Geometry check sheet. Reference: drawing and pictorial views, mm from the part's lowest x, y, z. A direction names the side the tool comes from. Round coordinates to 2 decimals unless told otherwise and drop trailing zeros. Write each loop counter-clockwise with the first axis right and the second up, starting at its lowest first coordinate (ties: lowest second). Pieces come first, ordered by that corner, then holes. Notation, with made-up numbers: M 32.25,-22.5 L 48.25,-22.5 A19 cw 48.25,3.5 Z; hole C -38.75,-30.75 d4. An arc over 180 degrees is marked long. Answer in a Markdown table with one row per item. Add a question column.
1. Sectioned sample at A-A on z = 18. Record the cut outline in (x, y).
2. Sectioned sample at B-B on y = 7.5. Record the cut outline in (x, z).
3. Sectioned sample at D-D on x = 38.5. Record the cut outline in (y, z).
4. Material ranges on probe 1 along Y at (x, z) = (37.5, 42.1); probe 2 along X at (y, z) = (7, 43.5) (1 decimal); probe 3 along Z at (x, y) = (29.5, 3.5), recorded low to high.
5. Go/stop test with flat-tipped pins: pin 1 Ø5.5 at (x, y) = (37.5, 7.5) entering from +Z; pin 2 Ø12 at (x, y) = (31.5, 21.5) entering from -Z; pin 3 Ø3 at (x, z) = (15, 31.5) entering from -Y; pin 4 Ø3 at (y, z) = (37.5, 14) entering from -X (1 decimal). Record where each tip stops, or that it passes through.
6. Draft check along X on the marked faces 1, 2 and 3. Enter one of: pulls with the +X half, pulls with the -X half, needs draft (parallel to the pull), parting line crosses it, or undercut.
7. Sectioned sample at C-C on x = 27. Record the cut outline in (y, z).
8. Set-up check for the marked faces 4 and 5: record each of +Z, -Z, +X, -X, +Y, -Y from which the full face is reachable in a straight line by a thin tool's end or side.
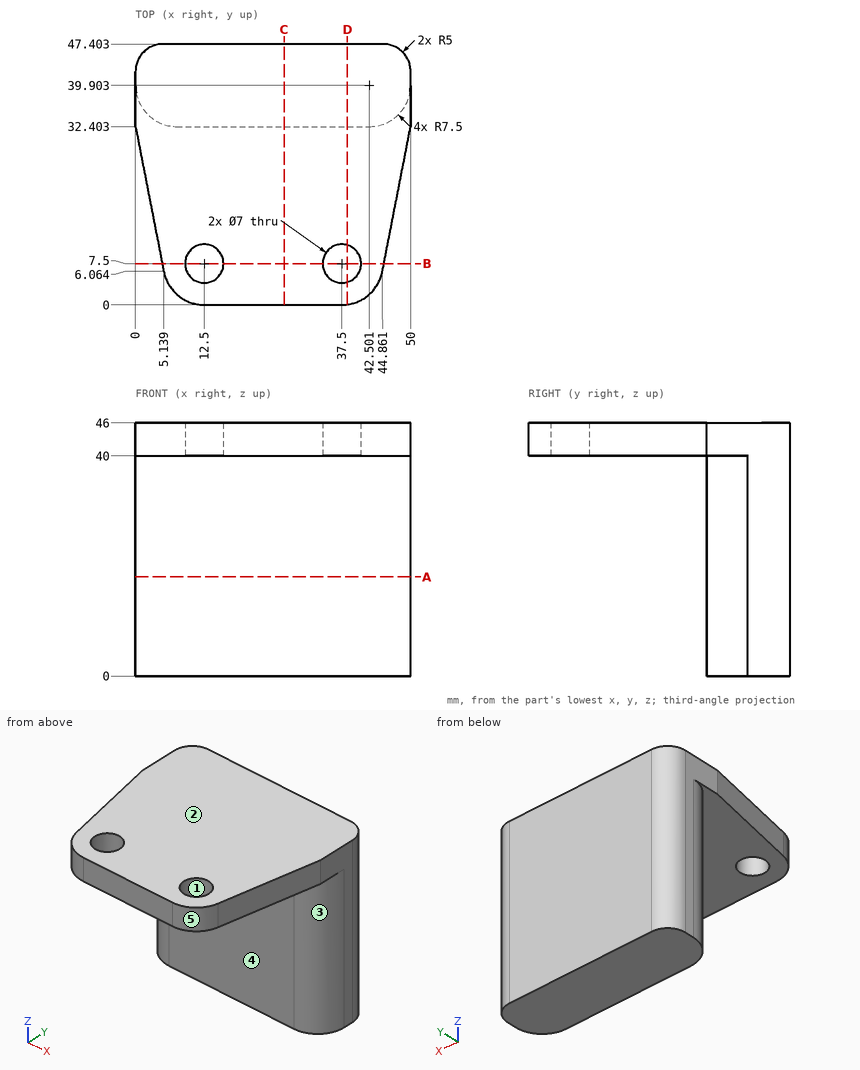
Geometry check:
| question | item | result |
|---|---|---|
| 1 | outline | M 0,39.9 A7.5 ccw 7.5,32.4 L 42.5,32.4 A7.5 ccw 50,39.81 L 50,42.4 A5 ccw 45,47.4 L 5,47.4 A5 ccw 0,42.4 Z |
| 2 | outline | M 4.86,40 L 9,40 L 9,46 L 4.86,46 Z; M 16,40 L 34,40 L 34,46 L 16,46 Z; M 41,40 L 45.14,40 L 45.14,46 L 41,46 Z |
| 3 | outline | M 0.07,40 L 4.15,40 L 4.15,46 L 0.07,46 Z; M 10.85,40 L 32.4,40 L 32.4,0 L 47.4,0 L 47.4,46 L 10.85,46 Z |
| 4 | probe 1 | y = 0 to 4, 11 to 47.4 |
| 4 | probe 2 | x = 5 to 9, 16 to 34, 41 to 45 |
| 4 | probe 3 | z = 40 to 46 |
| 5 | pin 1 | passes through |
| 5 | pin 2 | stops at z = 40 |
| 5 | pin 3 | stops at y = 32.4 |
| 5 | pin 4 | stops at x = 0.1 |
| 6 | face 1 | undercut |
| 6 | face 2 | needs draft |
| 6 | face 3 | pulls with the +X half |
| 7 | outline | M 0,40 L 32.4,40 L 32.4,0 L 47.4,0 L 47.4,46 L 0,46 Z |
| 8 | face 4 | -Z, +X, -X, -Y |
| 8 | face 5 | +Z, -Z, +X, -Y |
